Geometry: final body of the model. Coordinates: model frame, mm. A direction names the side the tool comes from. Give positions to 0.01 mm unless a question says otherwise; leave off trailing zeros. Write each loop counter-clockwise with the first axis right and the second up, starting at its lowest first coordinate (ties: lowest second). Pieces come first, ordered by that corner, then holes. Notation, with made-up numbers: (35.5, 60) - (63.5, 60) arc R31 cw to (63.5, 89) - close; hole circle Ø6 at (-34, 8.5). An arc over 180 degrees is marked (long way). Return JSON: item names as keys, results as strings.
from build123d import *

# Parameters (mm, degrees)
SKETCH1_R           = 6.35
BOSS_EXTRUDE2_DEPTH = 12.7
SKETCH2_R           = 6.35
BOSS_EXTRUDE3_DEPTH = 25.4


with BuildPart() as part:
    # Sketch1 → Boss-Extrude2 (new body)
    with BuildSketch(Plane.XY):
        with BuildLine():
            Line((72.806693362, 70.739109347), (-54.193306638, 70.739109347))
            Line((-54.193306638, 70.739109347), (-54.193306638, 13.589109347))
            Line((-54.193306638, 13.589109347), (72.806693362, 13.589109347))
            ThreePointArc((72.806693362, 13.589109347), (81.786949483, 17.308853226), (85.506693362, 26.289109347))
            Line((85.506693362, 26.289109347), (85.506693362, 58.039109347))
            ThreePointArc((85.506693362, 58.039109347), (81.786949483, 67.019365468), (72.806693362, 70.739109347))
        make_face()
        with Locations((72.806693362, 58.039109347)):
            Circle(SKETCH1_R, mode=Mode.SUBTRACT)
        with Locations((72.806693362, 26.289109347)):
            Circle(SKETCH1_R, mode=Mode.SUBTRACT)
    extrude(amount=BOSS_EXTRUDE2_DEPTH)

    # Sketch2 → Boss-Extrude3 (add)
    with BuildSketch(Plane.ZY.offset(54.193306638)):
        with BuildLine():
            Line((12.7, 13.589109347), (61.248819539, 30.143723397))
            ThreePointArc((61.248819539, 30.143723397), (69.85, 42.164109347), (61.248819539, 54.184495297))
            Line((61.248819539, 54.184495297), (12.7, 70.739109347))
            Line((12.7, 70.739109347), (12.7, 13.589109347))
        make_face()
        with Locations(Location((57.15, 42.164109347, 0), (0, 0, 270))):
            Circle(SKETCH2_R, mode=Mode.SUBTRACT)
    extrude(amount=-BOSS_EXTRUDE3_DEPTH)


solid = part.part
Q1. Section query B-B, the plane y = 62.5. Return the cut outline in (x, z), plus the area to 3 significant figures.
Answer key:
{"outline": "(-54.19, 0) - (68.29, 0) - (68.29, 12.7) - (-28.79, 12.7) - (-28.79, 36.86) - (-54.19, 36.86) - close; (77.33, 0) - (84.7, 0) - (84.7, 12.7) - (77.33, 12.7) - close", "area": "2,260 mm^2"}
Q2. Section query D-D, the plane z = 6. Return the cut outline in (x, y).
Answer key:
{"outline": "(-54.19, 13.59) - (72.81, 13.59) arc R12.7 ccw to (85.51, 26.29) - (85.51, 58.04) arc R12.7 ccw to (72.81, 70.74) - (-54.19, 70.74) - close; hole circle Ø12.7 at (72.81, 26.29); hole circle Ø12.7 at (72.81, 58.04)"}
Q3. Section query A-A, the plane x = -45. Return the cut outline in (y, z), plus the area to 3 significant figures.
Answer key:
{"outline": "(13.59, 0) - (70.74, 0) - (70.74, 12.7) - (54.18, 61.25) arc R12.7 ccw to (30.14, 61.25) - (13.59, 12.7) - close; hole circle Ø12.7 at (42.16, 57.15)", "area": "2,720 mm^2"}
Q4. Section query C-C, the plane z = 57.15. Return the cut outline in (x, y).
Answer key:
{"outline": "(-54.19, 28.75) - (-28.79, 28.75) - (-28.79, 35.81) - (-54.19, 35.81) - close; (-54.19, 48.51) - (-28.79, 48.51) - (-28.79, 55.58) - (-54.19, 55.58) - close"}
Q5. Set-up query: faces 1 (the flat face through (-28.793, 43, 35)), 2 (the flat face through (-41.67, 21.75, 36.63)). Return all of +Z, -Z, +X, -X, +Y, -Y with unobstructed straight access to the full face (end or side cutting, diameter ignored); none if empty.
Answer key:
{"face 1": "+Z, +X, +Y, -Y", "face 2": "+Z, +X, -X, -Y"}
Q6. Mould query, pull axis Y, two halves, no side actions, for faces 3 (the flat face through (15, 43, 0)), 4 (the cylindrical face through (81.885, 66.92, 6.261)), 5 (the cylindrical face through (78.672, 23.857, 6.261)). Classes: pulls with the +Y half, pulls with the -Y half, needs draft (parallel to the pull), parting line crosses it, or undercut.
Answer key:
{"face 3": "needs draft", "face 4": "pulls with the +Y half", "face 5": "undercut"}
Q7. Material intervals for probe 1 along Z at (x, y) = (-23, 45); probe 2 along X at (y, z) = (21.5, 13); probe 3 along Z at (x, y) = (-32, 39), sorted ascending. Write a range as [from, to].
Answer key:
{"probe 1": "z = [0, 12.7]", "probe 2": "x = [-54.19, -28.79]", "probe 3": "z = [0, 51.64], [62.66, 69.45]"}
Q8. Pin query (flat end, axial travel): P1, Ø1, axis at x = 66.5, y = 49.5, coming from the +Z side; P2, Ø17, axis at y = 29.5, z = 41.5, coming from the +X side. Return the tip coordinate at first contact, or that it passes through.
Answer key:
{"P1": "stops at z = 12.7", "P2": "stops at x = -28.79"}
